Source: three-view drawing plus pictorial views. Frame: mm from the lowest corner of the part. A direction names the side the tool comes from. Give positions to 0.01 mm unless a question says otherwise; leave off trailing zeros. Loops run counter-clockwise (first coordinate to the right, second up) from the corner with the lowest first, then second, coordinate; pieces in that order, holes last. Notation, with made-up numbers: (-16, 22.5) -> (38, 22.5) arc R34 cw to (38, 61.5) -> close; hole circle Ø4 at (-26, 4). An arc over 180 degrees is marked (long way). Put each result on its own line as item: value.
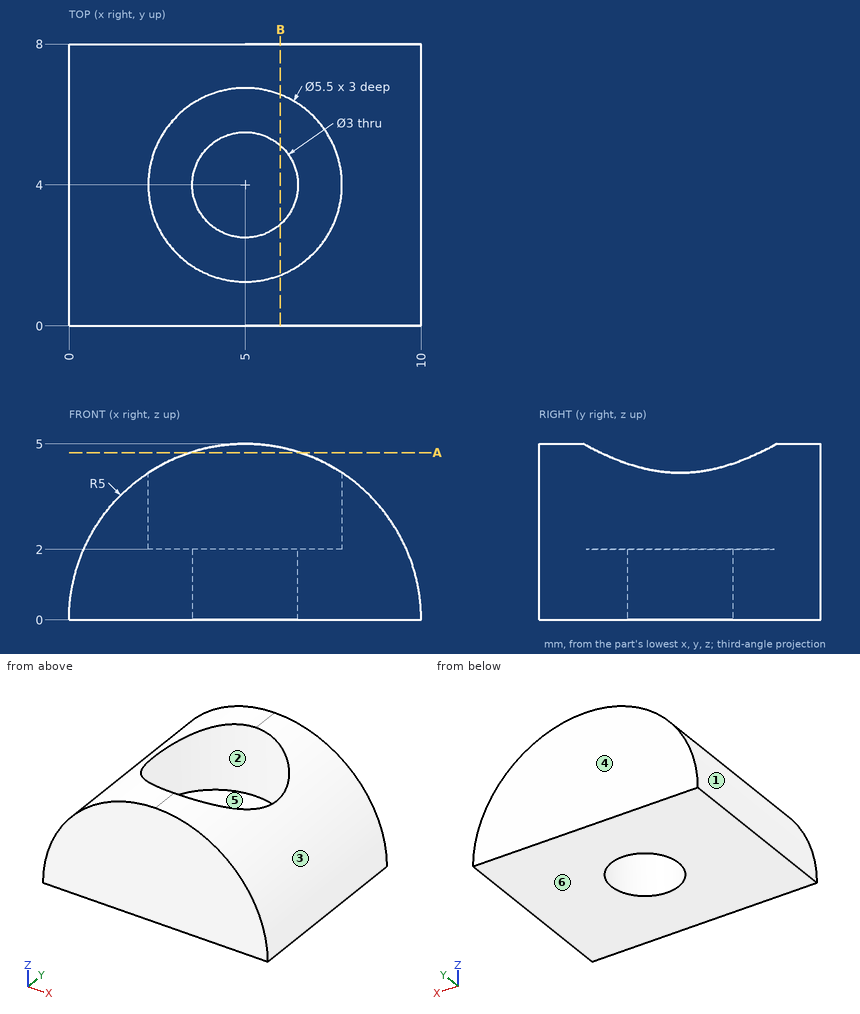
(1) Line query: probe 1 along Y at (x, z) = (5, 3.95); probe 2 along Z at (x, y) = (7.5, 4.75); probe 3 along X at (y, z) = (5, 2.25). Output: solid intervals per line, ascending. Write a range as from..to.
Calculated:
probe 1: y = 0..1.25, 6.75..8
probe 2: z = 0..2
probe 3: x = 0.53..2.44, 7.56..9.47
(2) Reachability of the marked faces 5 and 6 from +Z, -Z, +X, -X, +Y, -Y: full face, straight path, thin tool, end or side. Return the list, or none.
Calculated:
face 5: +Z
face 6: -Z, +X, -X, +Y, -Y
(3) Draft query along X for the marked faces 1, 2, 3 and 4. Return one class per face: released by +X, released by -X, zero draft, split by the parting line, or undercut.
Calculated:
face 1: released by -X
face 2: undercut
face 3: released by +X
face 4: zero draft
(4) First-contact query: P1, Ø1.6, axis at x = 5.5, y = 3, coming from the +Z side; P2, Ø2, axis at y = 2.5, z = 1.5, coming from the -X side. Flat tips, straight axial feed; report the tip coordinate or a pass-through.
Calculated:
P1: stops at z = 2
P2: stops at x = 0.03
(5) Section B-B on x = 6. Return loops of the section in (y, z), then the cut area to 3 significant figures.
Calculated:
outline: (0, 0) -> (2.88, 0) -> (2.88, 2) -> (1.44, 2) -> (1.44, 4.9) -> (0, 4.9) -> close; (5.12, 0) -> (8, 0) -> (8, 4.9) -> (6.56, 4.9) -> (6.56, 2) -> (5.12, 2) -> close
area: 19.9 mm²
(6) Section A-A on z = 4.75. Return loops of the section in (x, y), then the cut area to 3 significant figures.
Calculated:
outline: (3.44, 0) -> (6.56, 0) -> (6.56, 1.74) arc R2.75 cw to (3.44, 1.74) -> close; (3.44, 6.26) arc R2.75 cw to (6.56, 6.26) -> (6.56, 8) -> (3.44, 8) -> close
area: 8.78 mm²
